```python
from build123d import *

# Parameters (mm, degrees)
BOSS_EXTRUDE1_OUTLINE_R   = 558.8
BOSS_EXTRUDE1_OUTLINE_R_2 = 6.746875
BOSS_EXTRUDE1_OUTLINE_R_3 = 7
BOSS_EXTRUDE1_DEPTH       = 12.7
SKETCH2_R                 = 3.2639
CUT_EXTRUDE1_DEPTH        = 791.364580431


# Read off the part's stored shape, not the designer's step: Boss-Extrude1
with BuildPart() as part:
    # Boss-Extrude1 outline → Boss-Extrude1 (new body)
    with BuildSketch(Plane(origin=(0, 0, 0), x_dir=(1, 0, 0), z_dir=(0, 1, 0))):
        Circle(BOSS_EXTRUDE1_OUTLINE_R)
        with Locations((-337.806121582, -421.737177306)):
            Circle(BOSS_EXTRUDE1_OUTLINE_R_2, mode=Mode.SUBTRACT)
        with Locations((-296.708058268, -451.596668122)):
            Circle(BOSS_EXTRUDE1_OUTLINE_R_2, mode=Mode.SUBTRACT)
        with Locations((-25.4, -539.75)):
            Circle(BOSS_EXTRUDE1_OUTLINE_R_2, mode=Mode.SUBTRACT)
        with Locations((-263.157394541, -318.99201902)):
            Circle(BOSS_EXTRUDE1_OUTLINE_R_2, mode=Mode.SUBTRACT)
        with Locations((-222.059331227, -348.851509836)):
            Circle(BOSS_EXTRUDE1_OUTLINE_R_2, mode=Mode.SUBTRACT)
        with Locations((-25.4, -412.75)):
            Circle(BOSS_EXTRUDE1_OUTLINE_R_2, mode=Mode.SUBTRACT)
        with Locations((-25.4, -285.75)):
            Circle(BOSS_EXTRUDE1_OUTLINE_R_2, mode=Mode.SUBTRACT)
        with Locations((-505.483723013, -190.948758228)):
            Circle(BOSS_EXTRUDE1_OUTLINE_R_2, mode=Mode.SUBTRACT)
        with Locations((-521.181786327, -142.6350872)):
            Circle(BOSS_EXTRUDE1_OUTLINE_R_2, mode=Mode.SUBTRACT)
        with Locations((-384.699545444, -151.703599942)):
            Circle(BOSS_EXTRUDE1_OUTLINE_R_2, mode=Mode.SUBTRACT)
        with Locations((-400.397608758, -103.389928914)):
            Circle(BOSS_EXTRUDE1_OUTLINE_R_2, mode=Mode.SUBTRACT)
        with Locations((-279.613431188, -64.144770629)):
            Circle(BOSS_EXTRUDE1_OUTLINE_R_2, mode=Mode.SUBTRACT)
        with Locations((-147.410604185, -246.106351551)):
            Circle(BOSS_EXTRUDE1_OUTLINE_R_2, mode=Mode.SUBTRACT)
        with Locations((-188.5086675, -216.246860734)):
            Circle(BOSS_EXTRUDE1_OUTLINE_R_2, mode=Mode.SUBTRACT)
        with Locations((-158.038139321, -158.038139321)):
            Circle(BOSS_EXTRUDE1_OUTLINE_R_3, mode=Mode.SUBTRACT)
        with Locations((-85.529624675, -206.486779875)):
            Circle(BOSS_EXTRUDE1_OUTLINE_R_3, mode=Mode.SUBTRACT)
        with Locations((-263.915367874, -112.458441657)):
            Circle(BOSS_EXTRUDE1_OUTLINE_R_2, mode=Mode.SUBTRACT)
        with Locations((-206.486779875, -85.529624675)):
            Circle(BOSS_EXTRUDE1_OUTLINE_R_3, mode=Mode.SUBTRACT)
        with Locations((25.4, -539.75)):
            Circle(BOSS_EXTRUDE1_OUTLINE_R_2, mode=Mode.SUBTRACT)
        with Locations((25.4, -412.75)):
            Circle(BOSS_EXTRUDE1_OUTLINE_R_2, mode=Mode.SUBTRACT)
        with Locations((25.4, -285.75)):
            Circle(BOSS_EXTRUDE1_OUTLINE_R_2, mode=Mode.SUBTRACT)
        with Locations((222.059331227, -348.851509836)):
            Circle(BOSS_EXTRUDE1_OUTLINE_R_2, mode=Mode.SUBTRACT)
        with Locations((263.157394541, -318.99201902)):
            Circle(BOSS_EXTRUDE1_OUTLINE_R_2, mode=Mode.SUBTRACT)
        with Locations((296.708058268, -451.596668122)):
            Circle(BOSS_EXTRUDE1_OUTLINE_R_2, mode=Mode.SUBTRACT)
        with Locations((337.806121582, -421.737177306)):
            Circle(BOSS_EXTRUDE1_OUTLINE_R_2, mode=Mode.SUBTRACT)
        with Locations((0, -223.49968)):
            Circle(BOSS_EXTRUDE1_OUTLINE_R_3, mode=Mode.SUBTRACT)
        with Locations((85.529624675, -206.486779875)):
            Circle(BOSS_EXTRUDE1_OUTLINE_R_3, mode=Mode.SUBTRACT)
        with Locations((147.410604185, -246.106351551)):
            Circle(BOSS_EXTRUDE1_OUTLINE_R_2, mode=Mode.SUBTRACT)
        with Locations((188.5086675, -216.246860734)):
            Circle(BOSS_EXTRUDE1_OUTLINE_R_2, mode=Mode.SUBTRACT)
        with Locations((158.038139321, -158.038139321)):
            Circle(BOSS_EXTRUDE1_OUTLINE_R_3, mode=Mode.SUBTRACT)
        with Locations((206.486779875, -85.529624675)):
            Circle(BOSS_EXTRUDE1_OUTLINE_R_3, mode=Mode.SUBTRACT)
        with Locations((263.915367874, -112.458441657)):
            Circle(BOSS_EXTRUDE1_OUTLINE_R_2, mode=Mode.SUBTRACT)
        with Locations((384.699545444, -151.703599942)):
            Circle(BOSS_EXTRUDE1_OUTLINE_R_2, mode=Mode.SUBTRACT)
        with Locations((505.483723013, -190.948758228)):
            Circle(BOSS_EXTRUDE1_OUTLINE_R_2, mode=Mode.SUBTRACT)
        with Locations((521.181786327, -142.6350872)):
            Circle(BOSS_EXTRUDE1_OUTLINE_R_2, mode=Mode.SUBTRACT)
        with Locations((400.397608758, -103.389928914)):
            Circle(BOSS_EXTRUDE1_OUTLINE_R_2, mode=Mode.SUBTRACT)
        with Locations((279.613431188, -64.144770629)):
            Circle(BOSS_EXTRUDE1_OUTLINE_R_2, mode=Mode.SUBTRACT)
        with Locations((-279.613431188, 64.144770629)):
            Circle(BOSS_EXTRUDE1_OUTLINE_R_2, mode=Mode.SUBTRACT)
        with Locations((-400.397608758, 103.389928914)):
            Circle(BOSS_EXTRUDE1_OUTLINE_R_2, mode=Mode.SUBTRACT)
        with Locations((-521.181786327, 142.6350872)):
            Circle(BOSS_EXTRUDE1_OUTLINE_R_2, mode=Mode.SUBTRACT)
        with Locations((-505.483723013, 190.948758228)):
            Circle(BOSS_EXTRUDE1_OUTLINE_R_2, mode=Mode.SUBTRACT)
        with Locations((-384.699545444, 151.703599942)):
            Circle(BOSS_EXTRUDE1_OUTLINE_R_2, mode=Mode.SUBTRACT)
        with Locations((-223.49968, 0)):
            Circle(BOSS_EXTRUDE1_OUTLINE_R_3, mode=Mode.SUBTRACT)
        with Locations((-263.915367874, 112.458441657)):
            Circle(BOSS_EXTRUDE1_OUTLINE_R_2, mode=Mode.SUBTRACT)
        with Locations((-206.486779875, 85.529624675)):
            Circle(BOSS_EXTRUDE1_OUTLINE_R_3, mode=Mode.SUBTRACT)
        with Locations((-158.038139321, 158.038139321)):
            Circle(BOSS_EXTRUDE1_OUTLINE_R_3, mode=Mode.SUBTRACT)
        with Locations((-188.5086675, 216.246860734)):
            Circle(BOSS_EXTRUDE1_OUTLINE_R_2, mode=Mode.SUBTRACT)
        with Locations((-147.410604185, 246.106351551)):
            Circle(BOSS_EXTRUDE1_OUTLINE_R_2, mode=Mode.SUBTRACT)
        with Locations((-85.529624675, 206.486779875)):
            Circle(BOSS_EXTRUDE1_OUTLINE_R_3, mode=Mode.SUBTRACT)
        with Locations((-337.806121582, 421.737177306)):
            Circle(BOSS_EXTRUDE1_OUTLINE_R_2, mode=Mode.SUBTRACT)
        with Locations((-296.708058268, 451.596668122)):
            Circle(BOSS_EXTRUDE1_OUTLINE_R_2, mode=Mode.SUBTRACT)
        with Locations((-263.157394541, 318.99201902)):
            Circle(BOSS_EXTRUDE1_OUTLINE_R_2, mode=Mode.SUBTRACT)
        with Locations((-222.059331227, 348.851509836)):
            Circle(BOSS_EXTRUDE1_OUTLINE_R_2, mode=Mode.SUBTRACT)
        with Locations((-25.4, 285.75)):
            Circle(BOSS_EXTRUDE1_OUTLINE_R_2, mode=Mode.SUBTRACT)
        with Locations((-25.4, 412.75)):
            Circle(BOSS_EXTRUDE1_OUTLINE_R_2, mode=Mode.SUBTRACT)
        with Locations((-25.4, 539.75)):
            Circle(BOSS_EXTRUDE1_OUTLINE_R_2, mode=Mode.SUBTRACT)
        with BuildLine():
            ThreePointArc((10.995849972, 184.672930565), (0, -185), (-10.995849972, 184.672930565))
            ThreePointArc((-10.995849972, 184.672930565), (0, 196.00164), (10.995849972, 184.672930565))
        make_face(mode=Mode.SUBTRACT)
        with Locations((223.49968, 0)):
            Circle(BOSS_EXTRUDE1_OUTLINE_R_3, mode=Mode.SUBTRACT)
        with Locations((206.486779875, 85.529624675)):
            Circle(BOSS_EXTRUDE1_OUTLINE_R_3, mode=Mode.SUBTRACT)
        with Locations((263.915367874, 112.458441657)):
            Circle(BOSS_EXTRUDE1_OUTLINE_R_2, mode=Mode.SUBTRACT)
        with Locations((85.529624675, 206.486779875)):
            Circle(BOSS_EXTRUDE1_OUTLINE_R_3, mode=Mode.SUBTRACT)
        with Locations((0, 223.49968)):
            Circle(BOSS_EXTRUDE1_OUTLINE_R_3, mode=Mode.SUBTRACT)
        with Locations((158.038139321, 158.038139321)):
            Circle(BOSS_EXTRUDE1_OUTLINE_R_3, mode=Mode.SUBTRACT)
        with Locations((188.5086675, 216.246860734)):
            Circle(BOSS_EXTRUDE1_OUTLINE_R_2, mode=Mode.SUBTRACT)
        with Locations((147.410604185, 246.106351551)):
            Circle(BOSS_EXTRUDE1_OUTLINE_R_2, mode=Mode.SUBTRACT)
        with Locations((279.613431188, 64.144770629)):
            Circle(BOSS_EXTRUDE1_OUTLINE_R_2, mode=Mode.SUBTRACT)
        with Locations((400.397608758, 103.389928914)):
            Circle(BOSS_EXTRUDE1_OUTLINE_R_2, mode=Mode.SUBTRACT)
        with Locations((384.699545444, 151.703599942)):
            Circle(BOSS_EXTRUDE1_OUTLINE_R_2, mode=Mode.SUBTRACT)
        with Locations((521.181786327, 142.6350872)):
            Circle(BOSS_EXTRUDE1_OUTLINE_R_2, mode=Mode.SUBTRACT)
        with Locations((505.483723013, 190.948758228)):
            Circle(BOSS_EXTRUDE1_OUTLINE_R_2, mode=Mode.SUBTRACT)
        with Locations((25.4, 285.75)):
            Circle(BOSS_EXTRUDE1_OUTLINE_R_2, mode=Mode.SUBTRACT)
        with Locations((25.4, 412.75)):
            Circle(BOSS_EXTRUDE1_OUTLINE_R_2, mode=Mode.SUBTRACT)
        with Locations((222.059331227, 348.851509836)):
            Circle(BOSS_EXTRUDE1_OUTLINE_R_2, mode=Mode.SUBTRACT)
        with Locations((263.157394541, 318.99201902)):
            Circle(BOSS_EXTRUDE1_OUTLINE_R_2, mode=Mode.SUBTRACT)
        with Locations((25.4, 539.75)):
            Circle(BOSS_EXTRUDE1_OUTLINE_R_2, mode=Mode.SUBTRACT)
        with Locations((296.708058268, 451.596668122)):
            Circle(BOSS_EXTRUDE1_OUTLINE_R_2, mode=Mode.SUBTRACT)
        with Locations((337.806121582, 421.737177306)):
            Circle(BOSS_EXTRUDE1_OUTLINE_R_2, mode=Mode.SUBTRACT)
    extrude(amount=BOSS_EXTRUDE1_DEPTH)

    # Sketch2 → Cut-Extrude1 (cut, through all)
    with BuildSketch(Plane(origin=(0, 12.7, 0), x_dir=(1, 0, 0), z_dir=(0, 1, 0))):
        with Locations(Location((0, 508, 0), (0, 0, 270))):
            Circle(SKETCH2_R)
        with Locations(Location((-439.940905122, -254, 0), (0, 0, 270))):
            Circle(SKETCH2_R)
        with Locations(Location((439.940905122, -254, 0), (0, 0, 270))):
            Circle(SKETCH2_R)
    extrude(amount=-CUT_EXTRUDE1_DEPTH, mode=Mode.SUBTRACT)


solid = part.part
```
The listing builds one solid part. Answer for the finished solid, in the listing's coordinates (mm). Round coordinates to 2 decimals unless told otherwise and drop trailing zeros. Write each loop counter-clockwise with the first axis right and the second up, starting at its lowest first coordinate (ties: lowest second). Pieces come first, ordered by that corner, then holes. Notation, with made-up numbers: (15, 88.25) -> (26, 88.25) arc R12 cw to (26, 95.25) -> close; hole circle Ø3 at (5, 23.5). An arc over 180 degrees is marked (long way). Write item = value, one per line.
1) Section C-C on x = 317 is taken. Write down the section's boundary in (y, z), plus the area to 3 significant figures.
Check values:
outline = (0, -460.18) -> (12.7, -460.18) -> (12.7, 460.18) -> (0, 460.18) -> close
area = 11,700 mm²
2) Section B-B on y = 6.5 is taken. Give the number of separate pieces and of enclosed holes in the cut face, plus the area to 3 significant figures.
Check values:
separate_pieces = 1
enclosed_holes = 80
area = 862,000 mm²
3) Section A-A on x = 106 is taken. Write down the section's boundary in (y, z).
Check values:
outline = (0, -548.65) -> (12.7, -548.65) -> (12.7, -151.62) -> (0, -151.62) -> close; (0, 151.62) -> (12.7, 151.62) -> (12.7, 548.65) -> (0, 548.65) -> close
4) For a pull along Z with two mould halves and no side action, classify faces 1 (the cylindrical face through (7.98, 6.261, 184.828)), 2 (the cylindrical face through (-443.445, 6.261, 340.021)), 3 (the flat face through (-132, 12.7, -132)) as released by +Z, released by -Z, zero draft, split by the parting line, or undercut.
Check values:
face_1 = undercut
face_2 = split by the parting line
face_3 = zero draft
5) Section D-D on x = -459.5 is taken. Write down the section's boundary in (y, z), plus the area to 3 significant figures.
Check values:
outline = (0, -317.99) -> (12.7, -317.99) -> (12.7, 317.99) -> (0, 317.99) -> close
area = 8,080 mm²
6) Given pin 1 (22.5 mm diameter, centred on x = 0, z = 223.5, fed in from -Y); pin 2 (3 mm diameter, centred on y = 4, z = 378, fed in from +X); pin 3 (3 mm diameter, centred on x = 26.5, y = 3, fed in from +Z), each flat-ended and moving along its own axis, determine where each tip first touches the part or whether it passes through.
Check values:
pin_1 = 0
pin_2 = 412.92
pin_3 = 558.24
7) Straight lines are drawn through the part: line 1 along X through (y, z) = (2, -188); line 2 along X through (y, z) = (10, 411); line 3 along X through (y, z) = (5.75, 218). For each, find the intervals that lie inside material, in ascending order. Write a range as [from, to].
Check values:
line_1 = [-526.23, -511.55], [-499.42, -10.58], [10.58, 499.42], [511.55, 526.23]
line_2 = [-378.6, -31.92], [-18.88, 18.88], [31.92, 378.6]
line_3 = [-514.52, -195.02], [-181.99, -4.33], [4.33, 181.99], [195.02, 514.52]
